Work out the finished part from the listing and answer in its coordinate system (mm). Face numbers are marked on the shaded views. Round coordinates to 2 decimals unless told otherwise and drop trailing zeros. Order: outer loops, then holes, each group sorted by start corner. A loop starts at its lowest first (then second) coordinate and runs counter-clockwise, first axis right, second up. Notation, with made-up numbers: M -8,4.25 L 28,4.25 A19 ccw 28,40.25 Z; hole C -26,-38.5 d4. An arc over 180 degrees is marked long. Return JSON: item names as keys, results as strings.
from build123d import *

# Parameters (mm, degrees)
PAD_DEPTH    = 10
POCKET_DEPTH = 2
PAD001_DEPTH = 10
SKETCH002_R  = 2.75
HOLE_DEPTH   = 186.769494
FILLET_R     = 10


with BuildPart() as body:
    # Sketch → Pad (new body)
    with BuildSketch(Plane.XY):
        with BuildLine():
            ThreePointArc((50.827684, 0), (53.07085, 0.92915), (54, 3.172316))
            add(Edge.make_bspline(
                [(54, 3.172316), (53.770463, 24.754659), (48.332207, 42.658529)],
                knots=[0, 0, 0, 1, 1, 1], degree=2))
            add(Edge.make_bspline(
                [(48.332207, 42.658529), (47.508229, 44.694932), (42.952807, 43.870954), (38.691662, 46.837275), (36.784741, 50.827684)],
                knots=[0, 0, 0, 0, 0.5, 1, 1, 1, 1], degree=3))
            Line((36.784741, 50.827684), (0, 50.827684))
            Line((0, 50.827684), (0, 0))
            Line((0, 0), (50.827684, 0))
        make_face()
    pad = extrude(amount=PAD_DEPTH)

    # Mirrored: Pad across Sketch V_Axis
    add(pad.mirror(Plane(origin=(0, 0, 0), x_dir=(0, 0, 1), z_dir=(1, 0, 0))))

    # Sketch003 (on Face13 of Cut) → Pocket (cut)
    with BuildSketch(Plane.XY.offset(10)):
        with BuildLine():
            ThreePointArc((53.812202, 33.623601), (48.812202, 28.623601), (53.812202, 23.623601))
            Line((53.812202, 23.623601), (53.812202, 33.623601))
        make_face()
    pocket = extrude(amount=-POCKET_DEPTH, mode=Mode.SUBTRACT)

    # Mirrored003: Pocket across Sketch003 V_Axis
    add(pocket.mirror(Plane(origin=(0, 0, 10), x_dir=(0, 0, 1), z_dir=(1, 0, 0))), mode=Mode.SUBTRACT)


with BuildPart() as cut:
    # Sketch001 → Pad001 (new body)
    with BuildSketch(Plane.XY):
        Polygon((0, 0), (71.199806, 0), (71.199806, 6.985645), (59.457661, 6.985645), (50.704418, 53.954201), (0, 53.954201), align=None)
    pad001 = extrude(amount=PAD001_DEPTH)

    # Sketch002 (on Face3 of Pad001) → Hole (cut, through all)
    with BuildSketch(Plane(origin=(0, 6.985645, 0), x_dir=(-1, 0, 0), z_dir=(0, 1, 0))):
        with Locations((-65.328733, 5)):
            Circle(SKETCH002_R)
    hole = extrude(amount=-HOLE_DEPTH, mode=Mode.SUBTRACT)

    # Mirrored001: Pad001 across Sketch001 V_Axis
    add(pad001.mirror(Plane(origin=(0, 0, 0), x_dir=(0, 0, 1), z_dir=(1, 0, 0))))

    # Mirrored002: Hole across Sketch002 V_Axis
    add(hole.mirror(Plane(origin=(0, 6.985645, 0), x_dir=(0, 1, 0), z_dir=(-1, 0, 0))), mode=Mode.SUBTRACT)

    # Fillet
    fillet_edges = [cut.edges().sort_by_distance(p)[0] for p in [
        (50.704418, 53.954201, 5),
        (-50.704418, 53.954201, 5),
    ]]
    fillet(fillet_edges, radius=FILLET_R)

    # Cut: cut Body
    add(body.part, mode=Mode.SUBTRACT)


solid = cut.part
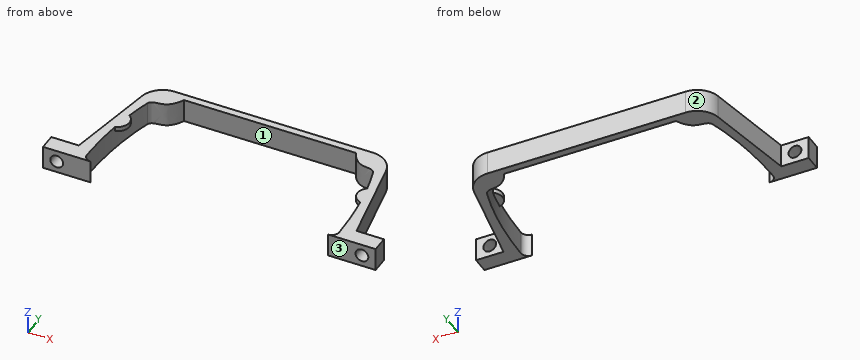
Item 1: Each of these flat-tipped pins is pushed along its axis until it touches: pin 1 (5 mm diameter, centred on x = -66, z = 4, fed in from +Y); pin 2 (5 mm diameter, centred on x = -9.5, z = 7.5, fed in from -Y); pin 3 (4 mm diameter, centred on y = 14.5, z = 8, fed in from +X). Where does it stop, or does it pass through?
Output:
{"pin 1": "stops at y = 6.99", "pin 2": "stops at y = 50.83", "pin 3": "stops at x = 58.43"}
Item 2: Consider line 1 along X through (y, z) = (26.5, 5.75); line 2 along X through (y, z) = (11, 1.5); line 3 along Y through (x, z) = (35, 9). Determine where each line is inside the solid, lowest interval first. Write a range as [from, to].
Output:
{"line 1": "x = [-55.82, -52.06], [52.06, 55.82]", "line 2": "x = [-58.71, -53.74], [53.74, 58.71]", "line 3": "y = [50.83, 53.95]"}
Item 3: The mould has two halves that part along X. Classify the marked faces 1, 2 and 3: pulls with the +X half, pulls with the -X half, needs draft (parallel to the pull), parting line crosses it, or undercut.
Output:
{"face 1": "undercut", "face 2": "pulls with the -X half", "face 3": "needs draft"}
Item 4: Find section B-B (z = 5). State how many separate pieces and enclosed holes the cut face has, plus the area to 3 significant figures.
Output:
{"separate pieces": "3", "enclosed holes": "0", "area": "939 mm^2"}
Item 5: Find section A-A (x = 2.5). Determine the outline of the cut face in (y, z).
Output:
{"outline": "M 50.83,0 L 53.95,0 L 53.95,10 L 50.83,10 Z"}
